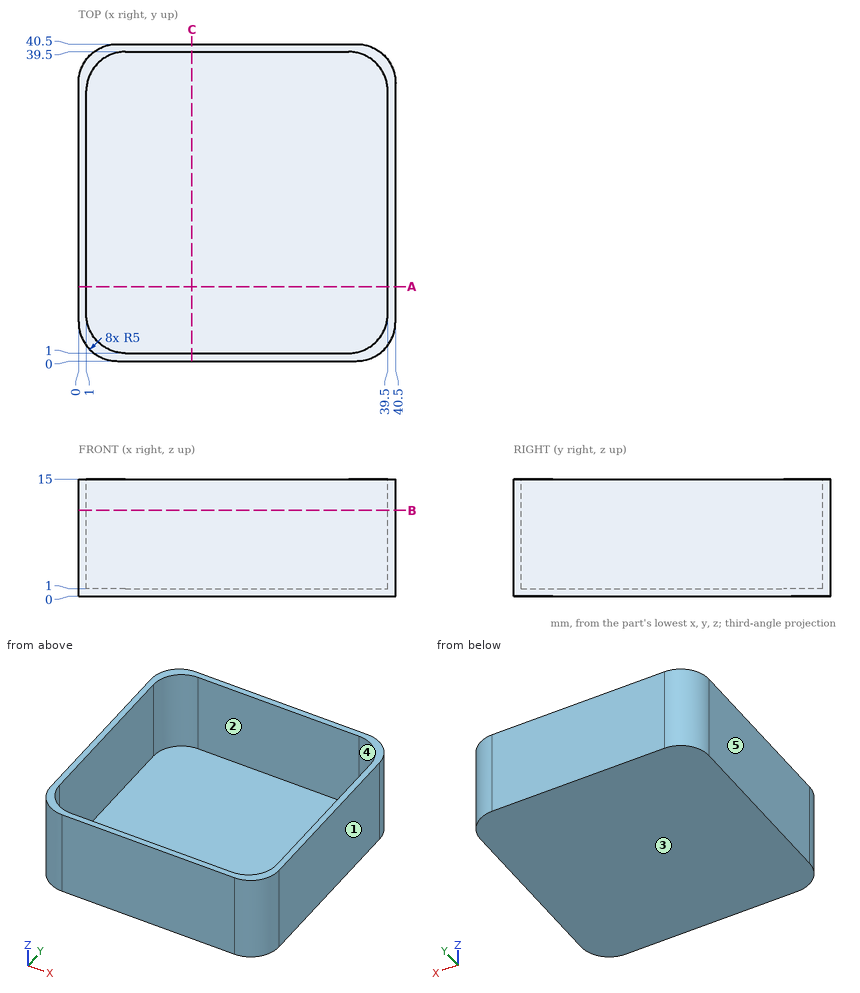
The figure shows three views and two pictorial views of one solid part (mm, origin at its lowest corner). Answer the questions. A direction names the side the tool comes from. Coordinates: 2 decimals unless noted, no trailing zeros. Loops run counter-clockwise (first coordinate to the right, second up) from the corner with the lowest first, then second, coordinate; pieces in that order, holes last. Notation, with made-up numbers: (46, 54) -> (61, 54) arc R16 cw to (61, 79) -> close; hole circle Ø3 at (-4.5, 5.5). An arc over 180 degrees is marked (long way). Use one line per item in the form item = value. Start each with the question number.
Item 1: A flat-ended cylindrical pin translates along its axis: pin 1 Ø11.5 at (x, y) = (29, 22.5) entering from +Z. Find the tip coordinate at first contact, or state that the pin passes through.
Item 2: The part is cut by section A-A on y = 9.5. Determine the outline of the cut face in (x, z).
Item 3: The mould has two halves that part along X. Classify the marked faces 3, 4 and 5: released by +X, released by -X, zero draft, split by the parting line, or undercut.
Item 4: The part is cut by section B-B on z = 11. Determine the outline of the cut face in (x, y), then the cut area to 3 significant figures.
Item 5: A tool of negligible diameter and unlimited length cuts with its end or side. For the marked faces 1 and 2, from which of +Z, -Z, +X, -X, +Y, -Y can it reach the whole face along a straight path? Write none if from no direction.
Item 6: Consider L1, parallel to Y at x = 13.5, z = 12.75; L2, parallel to Z at x = 8, y = 5. Determine where each line is inside the solid, lowest interval first. Write a range as [from, to].
Answer key:
q1.pin_1 = 1
q2.outline = (0, 0) -> (40.5, 0) -> (40.5, 15) -> (39.5, 15) -> (39.5, 1) -> (1, 1) -> (1, 15) -> (0, 15) -> close
q3.face_3 = zero draft
q3.face_4 = undercut
q3.face_5 = released by -X
q4.outline = (0, 5) arc R5 ccw to (5, 0) -> (35.5, 0) arc R5 ccw to (40.5, 5) -> (40.5, 35.5) arc R5 ccw to (35.5, 40.5) -> (5, 40.5) arc R5 ccw to (0, 35.5) -> close; hole (1, 6) arc R5 ccw to (6, 1) -> (34.5, 1) arc R5 ccw to (39.5, 6) -> (39.5, 34.5) arc R5 ccw to (34.5, 39.5) -> (6, 39.5) arc R5 ccw to (1, 34.5) -> close
q4.area = 158 mm2
q5.face_1 = +Z, -Z, +X, +Y, -Y
q5.face_2 = +Z
q6.L1 = [0, 1], [39.5, 40.5]
q6.L2 = [0, 1]
